```python
from build123d import *

# Parameters (mm, degrees)
NITROUS_BOSS_SKETCH_W          = 4
NITROUS_BOSS_SKETCH_H          = 7
ETHANOL_BOSS_SKETCH_W          = 4
ETHANOL_BOSS_SKETCH_H          = 7
CHAMBER_SKETCH_W               = 27.4
CHAMBER_SKETCH_H               = 5
FLAME_PASSAGE_SKETCH_W         = 16.5
FLAME_PASSAGE_SKETCH_H         = 1.5
PLUG_HOLE_SKETCH_W             = 9.6
PLUG_HOLE_SKETCH_H             = 4.5
NITROUS_SOCKET_SKETCH_W        = 1.6
NITROUS_SOCKET_SKETCH_H        = 7
NITROUS_ORIFICE_SKETCH_W       = 0.5
NITROUS_ORIFICE_SKETCH_H       = 2.5
ETHANOL_SOCKET_SKETCH_W        = 1.6
ETHANOL_SOCKET_SKETCH_H        = 7
ETHANOL_ORIFICE_SKETCH_W       = 0.5
ETHANOL_ORIFICE_SKETCH_H       = 2.5
NITROUS_SOCKET_RELIEF_SKETCH_W = 1.8
NITROUS_SOCKET_RELIEF_SKETCH_H = 1.5


with BuildPart() as part:
    # Body Sketch → Body (revolve)
    with BuildSketch(Plane.XY, mode=Mode.PRIVATE) as body_sk:
        Polygon((9.5, 0), (9.5, 4.953), (0, 4.953), (0, 9), (-42, 9), (-42, 0), align=None)
    revolve(body_sk.sketch.rotate(Axis((-300, 0, 0), (1, 0, 0)), 90), axis=Axis((-300, 0, 0), (1, 0, 0)))

    # Nitrous Boss Sketch → Nitrous Boss (revolve)
    with BuildSketch(Plane.XY, mode=Mode.PRIVATE) as nitrous_boss_sk:
        with Locations((-26, -9.5)):
            Rectangle(NITROUS_BOSS_SKETCH_W, NITROUS_BOSS_SKETCH_H)
    revolve(nitrous_boss_sk.sketch.rotate(Axis((-28, -3, 0), (0, -1, 0)), 90), axis=Axis((-28, -3, 0), (0, -1, 0)))

    # Ethanol Boss Sketch → Ethanol Boss (revolve)
    with BuildSketch(Plane(origin=(0, 0, 0), x_dir=(-1, 0, 0), z_dir=(0, -0.9169188892170476, 0.3990736155109426)), mode=Mode.PRIVATE) as ethanol_boss_sk:
        with Locations((30, -9.5)):
            Rectangle(ETHANOL_BOSS_SKETCH_W, ETHANOL_BOSS_SKETCH_H)
    revolve(ethanol_boss_sk.sketch.rotate(Axis((-32, 1.197220847, 2.750756668), (0, 0.39907361551094256, 0.9169188892170476)), 90), axis=Axis((-32, 1.197220847, 2.750756668), (0, 0.39907361551094256, 0.9169188892170476)))

    # Chamber Sketch → Chamber (revolve, cut)
    with BuildSketch(Plane.XY, mode=Mode.PRIVATE) as chamber_sk:
        with Locations((-19.7, 2.5)):
            Rectangle(CHAMBER_SKETCH_W, CHAMBER_SKETCH_H)
    revolve(chamber_sk.sketch.rotate(Axis((-300, 0, 0), (1, 0, 0)), 90), axis=Axis((-300, 0, 0), (1, 0, 0)), mode=Mode.SUBTRACT)

    # Flame Passage Sketch → Flame Passage (revolve, cut)
    with BuildSketch(Plane.XY, mode=Mode.PRIVATE) as flame_passage_sk:
        with Locations((2.25, 0.75)):
            Rectangle(FLAME_PASSAGE_SKETCH_W, FLAME_PASSAGE_SKETCH_H)
    revolve(flame_passage_sk.sketch.rotate(Axis((-300, 0, 0), (1, 0, 0)), 90), axis=Axis((-300, 0, 0), (1, 0, 0)), mode=Mode.SUBTRACT)

    # Plug Hole Sketch → Plug Hole (revolve, cut)
    with BuildSketch(Plane.XY, mode=Mode.PRIVATE) as plug_hole_sk:
        with Locations((-38.2, 2.25)):
            Rectangle(PLUG_HOLE_SKETCH_W, PLUG_HOLE_SKETCH_H)
    revolve(plug_hole_sk.sketch.rotate(Axis((-300, 0, 0), (1, 0, 0)), 90), axis=Axis((-300, 0, 0), (1, 0, 0)), mode=Mode.SUBTRACT)

    # Nitrous Socket Sketch → Nitrous Socket (revolve, cut)
    with BuildSketch(Plane.XY, mode=Mode.PRIVATE) as nitrous_socket_sk:
        with Locations((-27.2, -10.5)):
            Rectangle(NITROUS_SOCKET_SKETCH_W, NITROUS_SOCKET_SKETCH_H)
    revolve(nitrous_socket_sk.sketch.rotate(Axis((-28, -4, 0), (0, -1, 0)), 90), axis=Axis((-28, -4, 0), (0, -1, 0)), mode=Mode.SUBTRACT)

    # Nitrous Orifice Sketch → Nitrous Orifice (revolve, cut)
    with BuildSketch(Plane.XY, mode=Mode.PRIVATE) as nitrous_orifice_sk:
        with Locations((-27.75, -5.75)):
            Rectangle(NITROUS_ORIFICE_SKETCH_W, NITROUS_ORIFICE_SKETCH_H)
    revolve(nitrous_orifice_sk.sketch.rotate(Axis((-28, -1.5, 0), (0, -1, 0)), 90), axis=Axis((-28, -1.5, 0), (0, -1, 0)), mode=Mode.SUBTRACT)

    # Ethanol Socket Sketch → Ethanol Socket (revolve, cut)
    with BuildSketch(Plane(origin=(0, 0, 0), x_dir=(-1, 0, 0), z_dir=(0, -0.9169188892170476, 0.3990736155109426)), mode=Mode.PRIVATE) as ethanol_socket_sk:
        with Locations((31.2, -10.5)):
            Rectangle(ETHANOL_SOCKET_SKETCH_W, ETHANOL_SOCKET_SKETCH_H)
    revolve(ethanol_socket_sk.sketch.rotate(Axis((-32, 1.596294462, 3.667675557), (0, 0.39907361551094267, 0.9169188892170476)), 90), axis=Axis((-32, 1.596294462, 3.667675557), (0, 0.39907361551094267, 0.9169188892170476)), mode=Mode.SUBTRACT)

    # Ethanol Orifice Sketch → Ethanol Orifice (revolve, cut)
    with BuildSketch(Plane(origin=(0, 0, 0), x_dir=(-1, 0, 0), z_dir=(0, -0.9169188892170476, 0.3990736155109426)), mode=Mode.PRIVATE) as ethanol_orifice_sk:
        with Locations((31.75, -5.75)):
            Rectangle(ETHANOL_ORIFICE_SKETCH_W, ETHANOL_ORIFICE_SKETCH_H)
    revolve(ethanol_orifice_sk.sketch.rotate(Axis((-32, 0.598610423, 1.375378334), (0, 0.39907361551094256, 0.9169188892170476)), 90), axis=Axis((-32, 0.598610423, 1.375378334), (0, 0.39907361551094256, 0.9169188892170476)), mode=Mode.SUBTRACT)

    # Nitrous Socket Relief Sketch → Nitrous Socket Relief (revolve, cut)
    with BuildSketch(Plane.XY, mode=Mode.PRIVATE) as nitrous_socket_relief_sk:
        with Locations((-27.1, -13.25)):
            Rectangle(NITROUS_SOCKET_RELIEF_SKETCH_W, NITROUS_SOCKET_RELIEF_SKETCH_H)
    revolve(nitrous_socket_relief_sk.sketch.rotate(Axis((-28, -18, 0), (0, 1, 0)), 270), axis=Axis((-28, -18, 0), (0, 1, 0)), mode=Mode.SUBTRACT)


solid = part.part
```
Build history of the part. All positions in model axes, mm. A direction names the side the tool comes from. Give positions to 0.01 mm unless a question says otherwise; leave off trailing zeros. Loops run counter-clockwise (first coordinate to the right, second up) from the corner with the lowest first, then second, coordinate; pieces in that order, holes last. Notation, with made-up numbers: (-23, -13.75) -> (9, -13.75) arc R8 ccw to (9, -5.75) -> close; hole circle Ø10 at (2.25, -9.5). An arc over 180 degrees is marked (long way). One line per question, with ' | ' between items.
Q1. Drill centre lines: line 1 along X through (y, z) = (-9.85, 0); line 2 along Z through (x, y) = (-28, -8.5); line 3 along X through (y, z) = (2.5, -4). Where is each one in solid material? Low to high. Write a range as [from, to].
Filled sheet:
line 1: x = [-32, -29.6], [-26.4, -24] | line 2: z = [-4, -1.6], [1.6, 4] | line 3: x = [-42, -33.4], [-6, 9.5]
Q2. Cut at B-B, the plane x = 3. Write the cut outline in (y, z), plus the area to 3 significant figures.
Filled sheet:
outline: circle Ø9.91 at (0, 0); hole circle Ø3 at (0, 0) | area: 70.0 mm²
Q3. Tool access for faces 5 (the flat face through (0, 4, -4)), 6 (the cylindrical face through (-29.586, -9.712, -0.208)), 7 (the flat face through (-6, -1.2, 1.2)): list every direction of +Z, -Z, +X, -X, +Y, -Y with a clear straight run to the whole face (end or side of a thin tool).
Filled sheet:
face 5: +X | face 6: -Y | face 7: none
Q4. Pull direction Y, two halves, no side cores. Call faces 1 (the flat face through (-30, 5, 12)), 2 (the flat face through (-27, -13, -2)), 3 (the flat face through (9.5, -1.2, 1.2)), 4 (the cylindrical face through (1.86, -0.45, 1.43)): pulls with the +Y half, pulls with the -Y half, needs draft (parallel to the pull), parting line crosses it, or undercut.
Filled sheet:
face 1: pulls with the +Y half | face 2: pulls with the -Y half | face 3: needs draft | face 4: undercut
Q5. Cut at C-C, the plane z = 2.5. Write the cut outline in (x, y).
Filled sheet:
outline: (-42, -8.65) -> (-31.12, -8.65) -> (-31.12, -13) -> (-24.88, -13) -> (-24.88, -8.65) -> (0, -8.65) -> (0, -4.28) -> (9.5, -4.28) -> (9.5, 4.28) -> (0, 4.28) -> (0, 8.65) -> (-42, 8.65) -> (-42, 3.74) -> (-33.4, 3.74) -> (-33.4, 4.33) -> (-6, 4.33) -> (-6, -4.33) -> (-33.4, -4.33) -> (-33.4, -3.74) -> (-42, -3.74) -> close
Q6. Cut at D-D, the plane y = -2.5. Write the cut outline in (x, z), plus the area to 3 significant figures.
Filled sheet:
outline: (-42, -8.65) -> (0, -8.65) -> (0, -4.28) -> (9.5, -4.28) -> (9.5, 4.28) -> (0, 4.28) -> (0, 8.65) -> (-42, 8.65) -> (-42, 3.74) -> (-33.4, 3.74) -> (-33.4, 4.33) -> (-6, 4.33) -> (-6, -4.33) -> (-33.4, -4.33) -> (-33.4, -3.74) -> (-42, -3.74) -> close | area: 506 mm²
Q7. Drop flat-ended pins along their axis: pin 1 (8 mm diameter, centred on y = -0.5, z = 11, fed in from +X); pin 2 (2 mm diameter, centred on x = -16, y = -6, fed in from -Z); pin 3 (4 mm diameter, centred on y = 6, z = 10.5, fed in from +X). Give the stop position or say it passes through.
Filled sheet:
pin 1: stops at x = 0 | pin 2: stops at z = -7.48 | pin 3: stops at x = -28
Q8. Cut at A-A, the plane z = 0. Count the separate pieces of the cut face and the enclosed holes in it, plus the area to 3 significant figures.
Filled sheet:
separate pieces: 3 | enclosed holes: 0 | area: 463 mm²
